from build123d import *

# Parameters (mm, degrees)
SKETCH1_W                = 50
SKETCH1_H                = 50
BOSS_EXTRUDE1_DEPTH      = 2
M3_CLEARANCE_HOLE1_D     = 3.2
M3_CLEARANCE_HOLE2_D     = 3
M2_CLEARANCE_HOLE1_D     = 2
M2_CLEARANCE_HOLE1_DEPTH = 10
M2_CLEARANCE_HOLE1_TIP   = 0.600860619


with BuildPart() as part:
    # Sketch1 → Boss-Extrude1 (new body)
    with BuildSketch(Plane(origin=(0, 0, 0), x_dir=(1, 0, 0), z_dir=(0, 1, 0))):
        with Locations((25, 25)):
            Rectangle(SKETCH1_W, SKETCH1_H)
    extrude(amount=BOSS_EXTRUDE1_DEPTH)

    # M3 Clearance Hole1 (through all)
    with Locations(Plane(origin=(0, 2, 0), x_dir=(1, 0, 0), z_dir=(0, 1, 0))):
        with Locations((2.5, 2.5)):
            Hole(M3_CLEARANCE_HOLE1_D / 2)

    # M3 Clearance Hole2 (through all)
    with Locations(Plane(origin=(0, 2, 0), x_dir=(1, 0, 0), z_dir=(0, 1, 0))):
        with Locations((47.5, 2.5), (47.5, 47.5), (2.5, 47.5)):
            Hole(M3_CLEARANCE_HOLE2_D / 2)

    # M2 Clearance Hole1
    with Locations(Plane(origin=(0, 2, 0), x_dir=(1, 0, 0), z_dir=(0, 1, 0))):
        with Locations((3, 10), (3, 40), (47, 40), (47, 10)):
            Hole(M2_CLEARANCE_HOLE1_D / 2, depth=M2_CLEARANCE_HOLE1_DEPTH)
            with Locations((0, 0, -(M2_CLEARANCE_HOLE1_DEPTH + M2_CLEARANCE_HOLE1_TIP / 2))):  # 118° drill point
                Cone(0, M2_CLEARANCE_HOLE1_D / 2, M2_CLEARANCE_HOLE1_TIP, mode=Mode.SUBTRACT)


solid = part.part
Verification items for the finished model (mm, model axes). Coordinates: 2 decimals unless noted, no trailing zeros. Order: outer loops, then holes, each group sorted by start corner. A loop starts at its lowest first (then second) coordinate and runs counter-clockwise, first axis right, second up. Notation, with made-up numbers: M 48,71.25 L 62,71.25 A24 cw 62,93.25 Z; hole C -2.5,-18 d5. An arc over 180 degrees is marked long. One line per item, written item: value. Start each with the question number.
Item 1: Sectioned sample at A-A (z = -40). Enter the section's corners in (x, y), then the cut area to 3 significant figures.
Item 2: Scan lines: probe 1 along X at (y, z) = (1.25, -40); probe 2 along Z at (x, y) = (47, 0.4); probe 3 along X at (y, z) = (1, -9.5). Record each from-to range of solid material in increasing order.
Item 3: Sectioned sample at D-D (z = -2.5). Enter the section's corners in (x, y), then the cut area to 3 significant figures.
Item 4: Sectioned sample at C-C (x = 47). Enter the section's corners in (y, z).
Item 5: Sectioned sample at B-B (y = 1.3). Count the separate pieces of the cut face and the enclosed holes in it, then the cut area to 3 significant figures.
Item 6: Mould release check, pull along X, two halves, no side actions. Record for faces 1 (the flat face through (0, 1, -25)), 2 (the cylindrical face through (3, 1, -41)), 3 (the flat face through (25, 0, -25)): released by +X, released by -X, zero draft, split by the parting line, or undercut.
Conclusion:
1. outline: M 0,0 L 2,0 L 2,2 L 0,2 Z; M 4,0 L 46,0 L 46,2 L 4,2 Z; M 48,0 L 50,0 L 50,2 L 48,2 Z
1. area: 92.0 mm^2
2. probe 1: x = 0 to 2, 4 to 46, 48 to 50
2. probe 2: z = -50 to -48.91, -46.09 to -41, -39 to -11, -9 to -3.91, -1.09 to 0
2. probe 3: x = 0 to 2.13, 3.87 to 46.13, 47.87 to 50
3. outline: M 0,0 L 0.9,0 L 0.9,2 L 0,2 Z; M 4.1,0 L 46,0 L 46,2 L 4.1,2 Z; M 49,0 L 50,0 L 50,2 L 49,2 Z
3. area: 87.6 mm^2
4. outline: M 0,-50 L 2,-50 L 2,-48.91 L 0,-48.91 Z; M 0,-46.09 L 2,-46.09 L 2,-41 L 0,-41 Z; M 0,-39 L 2,-39 L 2,-11 L 0,-11 Z; M 0,-9 L 2,-9 L 2,-3.91 L 0,-3.91 Z; M 0,-1.09 L 2,-1.09 L 2,0 L 0,0 Z
5. separate pieces: 1
5. enclosed holes: 8
5. area: 2,460 mm^2
6. face 1: released by -X
6. face 2: undercut
6. face 3: zero draft
